```python
from build123d import *

# Parameters (mm, degrees)
SKETCH1_W           = 1120
SKETCH1_H           = 730
BOSS_EXTRUDE2_DEPTH = 1.5


with BuildPart() as part:
    # Sketch1 → Boss-Extrude2 (new body)
    with BuildSketch(Plane.XY):
        Rectangle(SKETCH1_W, SKETCH1_H)
        with BuildLine():
            Line((250, 195.535714286), (-250, 195.535714286))
            ThreePointArc((-250, 195.535714286), (-285.355339059, 180.891053345), (-300, 145.535714286))
            Line((-300, 145.535714286), (-300, -145.535714286))
            ThreePointArc((-300, -145.535714286), (-285.355339059, -180.891053345), (-250, -195.535714286))
            Line((-250, -195.535714286), (250, -195.535714286))
            ThreePointArc((250, -195.535714286), (285.355339059, -180.891053345), (300, -145.535714286))
            Line((300, -145.535714286), (300, 145.535714286))
            ThreePointArc((300, 145.535714286), (285.355339059, 180.891053345), (250, 195.535714286))
        make_face(mode=Mode.SUBTRACT)
    extrude(amount=BOSS_EXTRUDE2_DEPTH)


solid = part.part
```
The model under review builds one solid part; all positions refer to its coordinate system, in mm. A direction names the side the tool comes from. Give positions to 0.01 mm unless a question says otherwise; leave off trailing zeros. Write each loop counter-clockwise with the first axis right and the second up, starting at its lowest first coordinate (ties: lowest second). Pieces come first, ordered by that corner, then holes. Notation, with made-up numbers: (78, -26.5) -> (82, -26.5) arc R23 cw to (82, 8.5) -> close; hole circle Ø11 at (77, 22.5). An arc over 180 degrees is marked (long way). Put each result on its own line as item: value.
(1) We need section C-C, the plane y = 119. Give the boundary of the cut face in (x, z), and give its area (3 significant figures).
Results are:
outline: (-560, 0) -> (-300, 0) -> (-300, 1.5) -> (-560, 1.5) -> close; (300, 0) -> (560, 0) -> (560, 1.5) -> (300, 1.5) -> close
area: 780 mm²
(2) We need section A-A, the plane x = 27. Give the boundary of the cut face in (y, z).
Results are:
outline: (-365, 0) -> (-195.54, 0) -> (-195.54, 1.5) -> (-365, 1.5) -> close; (195.54, 0) -> (365, 0) -> (365, 1.5) -> (195.54, 1.5) -> close
(3) For pin 1 Ø3 at (x, y) = (348, 222) entering from -Z, flat-tipped, find the tip position at first contact; note if it passes through.
Results are:
pin 1: z = 0
(4) To check wall thickness, follow probe 1 along X at (y, z) = (-47, 0.55); probe 2 along Y at (x, z) = (0.5, 1.4); probe 3 along X at (y, z) = (-154, 1). State the ranges of each line that lie inside material, in increasing order. Write a range as from..to.
Results are:
probe 1: -560..-300, 300..560
probe 2: -365..-195.54, 195.54..365
probe 3: -560..-299.28, 299.28..560
(5) Tool access review of faces 4 (the flat face through (-8, 248, 1.5)), 5 (the cylindrical face through (-285.74, -180.5, 0.74)): name each direction out of +Z, -Z, +X, -X, +Y, -Y from which nothing blocks a thin tool from reaching the whole face with its end or side.
Results are:
face 4: +Z, +X, -X, +Y, -Y
face 5: +Z, -Z
(6) We need section B-B, the plane z = 1.1. Give the boundary of the cut face in (x, y), and give its area (3 significant figures).
Results are:
outline: (-560, -365) -> (560, -365) -> (560, 365) -> (-560, 365) -> close; hole (-300, -145.54) arc R50 ccw to (-250, -195.54) -> (250, -195.54) arc R50 ccw to (300, -145.54) -> (300, 145.54) arc R50 ccw to (250, 195.54) -> (-250, 195.54) arc R50 ccw to (-300, 145.54) -> close
area: 585,000 mm²
(7) The part is to be moulded in two halves that separate along X. For faces 1 (the cylindrical face through (284.96, -181.28, 0.74)), 2 (the flat face through (-8, 248, 0)), 3 (the cylindrical face through (-284.96, 181.28, 0.74)), say which applies: pulls with the +X half, pulls with the -X half, needs draft (parallel to the pull), parting line crosses it, or undercut.
Results are:
face 1: undercut
face 2: needs draft
face 3: undercut
